Design review of the part built by this model. Coordinates are the model's own, in mm. Coordinates: 2 decimals unless noted, no trailing zeros. Order: outer loops, then holes, each group sorted by start corner. A loop starts at its lowest first (then second) coordinate and runs counter-clockwise, first axis right, second up. Notation, with made-up numbers: M -20.75,78 L 10.25,78 A6 cw 10.25,82 Z; hole C 21.5,64.25 d3. An arc over 180 degrees is marked long. Answer as a JSON object with one key per item and string values.
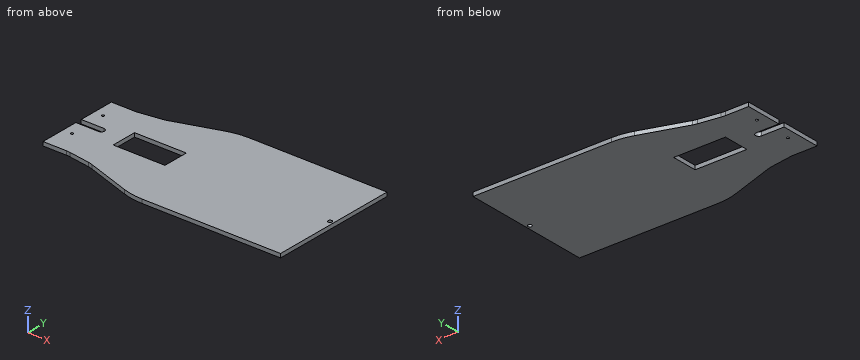
from build123d import *

# Parameters (mm, degrees)
RESSALTO_EXTRUS_O2_DEPTH = 3
FILETE4_R                = 50
FILETE6_R                = 20
ESBO_O3_R                = 1.000396488
CORTE_EXTRUS_O1_DEPTH    = 3
ESBO_O4_R                = 2.5
CORTE_EXTRUS_O3_DEPTH    = 3
ESBO_O5_R                = 1
CORTE_EXTRUS_O4_DEPTH    = 3
ESBO_O6_W                = 28
ESBO_O6_H                = 99.656129788
CORTE_EXTRUS_O5_DEPTH    = 10
ESBO_O7_R                = 1.5
CORTE_EXTRUS_O6_DEPTH    = 10
ESBO_O8_W                = 40
ESBO_O8_H                = 20
CORTE_EXTRUS_O7_DEPTH    = 10


with BuildPart() as part:
    # Esboço1 → Ressalto-extrusão2 (new body)
    with BuildSketch(Plane.XY):
        Polygon((130.267029072, 60.684036759), (130.267029072, -38.972093029), (-12.814839489, -38.972093029), (-57.051670623, -24.075187779), (-76.551670623, -21.075187779), (-96.051670623, -21.075187779), (-96.051670623, -19.075187779), (-96.051670623, 10.924812221), (-96.051670623, 40.924812221), (-96.051670623, 42.924812221), (-76.551670623, 42.924812221), (-57.051670623, 45.924812221), (-12.66677951, 60.684036759), align=None)
    extrude(amount=RESSALTO_EXTRUS_O2_DEPTH)

    # Filete4
    filete4_edges = [part.edges().sort_by_distance(p)[0] for p in [
        (-12.814839489, -38.972093029, 1.5),
        (-12.66677951, 60.684036759, 1.5),
    ]]
    fillet(filete4_edges, radius=FILETE4_R)

    # Filete6
    filete6_edges = [part.edges().sort_by_distance(p)[0] for p in [
        (-57.051670623, -24.075187779, 1.5),
        (-76.551670623, -21.075187779, 1.5),
        (-76.551670623, 42.924812221, 1.5),
        (-57.051670623, 45.924812221, 1.5),
    ]]
    fillet(filete6_edges, radius=FILETE6_R)

    # Esboço3 → Corte-extrusão1 (cut)
    with BuildSketch(Plane.XY.offset(3)):
        with Locations((127.267029072, 10.855971865)):
            Circle(ESBO_O3_R)
    extrude(amount=-CORTE_EXTRUS_O1_DEPTH, mode=Mode.SUBTRACT)

    # Esboço4 → Corte-extrusão3 (cut)
    with BuildSketch(Plane.XY.offset(3)):
        with BuildLine():
            Line((-78.551670623, 14.705809502), (-96.051670623, 14.705809502))
            Line((-96.051670623, 14.705809502), (-96.051670623, 12.205809502))
            Line((-96.051670623, 12.205809502), (-81.051670623, 12.205809502))
            ThreePointArc((-81.051670623, 12.205809502), (-80.319437576, 13.973576455), (-78.551670623, 14.705809502))
        make_face()
        with BuildLine():
            Line((-81.051670623, 12.205809502), (-96.051670623, 12.205809502))
            Line((-96.051670623, 12.205809502), (-96.051670623, 9.705809502))
            Line((-96.051670623, 9.705809502), (-78.551670623, 9.705809502))
            ThreePointArc((-78.551670623, 9.705809502), (-80.319437576, 10.438042549), (-81.051670623, 12.205809502))
        make_face()
        with Locations((-78.551670623, 12.205809502)):
            Circle(ESBO_O4_R)
    extrude(amount=-CORTE_EXTRUS_O3_DEPTH, mode=Mode.SUBTRACT)

    # Esboço5 → Corte-extrusão4 (cut)
    with BuildSketch(Plane.XY.offset(3)):
        with Locations((-89.059378868, -2.294160789)):
            Circle(ESBO_O5_R)
        with Locations((-89.102120748, 26.704536083)):
            Circle(ESBO_O5_R)
    extrude(amount=-CORTE_EXTRUS_O4_DEPTH, mode=Mode.SUBTRACT)

    # Esboço6 → Corte-extrusão5 (cut)
    with BuildSketch(Plane.XY.offset(3)):
        with Locations((116.267029072, 10.855971865)):
            Rectangle(ESBO_O6_W, ESBO_O6_H)
    extrude(amount=-CORTE_EXTRUS_O5_DEPTH, mode=Mode.SUBTRACT)

    # Esboço7 → Corte-extrusão6 (cut)
    with BuildSketch(Plane.XY.offset(3)):
        with Locations((99.400721929, 10.855971865)):
            Circle(ESBO_O7_R)
    extrude(amount=-CORTE_EXTRUS_O6_DEPTH, mode=Mode.SUBTRACT)

    # Esboço8 → Corte-extrusão7 (cut)
    with BuildSketch(Plane.XY.offset(3)):
        with Locations((-41.051670623, 12.205809502)):
            Rectangle(ESBO_O8_W, ESBO_O8_H)
    extrude(amount=-CORTE_EXTRUS_O7_DEPTH, mode=Mode.SUBTRACT)


solid = part.part
1) To check wall thickness, follow L1, parallel to Y at x = -87, z = 2.45; L2, parallel to X at y = 9, z = 0.9; L3, parallel to Y at x = -59, z = 1.7. State the ranges of each line that lie inside material, in increasing order.
Taken from the geometry:
{"L1": "y = -21.08 to 9.71, 14.71 to 42.92", "L2": "x = -96.05 to -61.05, -21.05 to 102.27", "L3": "y = -23.78 to 2.21, 22.21 to 45.63"}
2) Add section A-A (z = 2.25). State the section outline as (x, y) points, and give its area (3 significant figures).
Taken from the geometry:
{"outline": "M -96.05,-21.08 L -78.08,-21.08 A20 cw -75.04,-21.31 L -58.76,-23.81 A20 cw -55.42,-24.63 L -20.58,-36.36 A50 ccw -4.62,-38.97 L 102.27,-38.97 L 102.27,60.68 L -4.57,60.68 A50 ccw -20.35,58.13 L -55.45,46.46 A20 cw -58.72,45.67 L -75.04,43.16 A20 cw -78.08,42.92 L -96.05,42.92 L -96.05,14.71 L -78.55,14.71 A2.5 cw -78.55,9.71 L -96.05,9.71 Z; hole C -89.1,26.7 d2; hole C -89.06,-2.29 d2; hole M -61.05,2.21 L -21.05,2.21 L -21.05,22.21 L -61.05,22.21 Z; hole C 99.4,10.86 d3", "area": "16,900 mm2"}
3) Insertion check: pin 1 Ø1 at (x, z) = (-41, 2) entering from +Y; pin 2 Ø5 at (x, y) = (99.4, 10.86) entering from -Z; pin 3 Ø1.5 at (x, z) = (-91, 2) entering from -Y; pin 4 Ø1.5 at (x, z) = (-86.5, 1) entering from +Y. Each pin has a flat end and moves straight along its axis. Give the tip position at first contact, or say it passes through.
Taken from the geometry:
{"pin 1": "stops at y = 51.43", "pin 2": "stops at z = 0", "pin 3": "stops at y = -21.08", "pin 4": "stops at y = 42.92"}
